```python
from build123d import *

# Parameters (mm, degrees)
SKETCH1_W           = 27.5
SKETCH1_H           = 32.4
BOSS_EXTRUDE1_DEPTH = 1.6
SKETCH2_W           = 18.4
SKETCH2_H           = 13.4
BOSS_EXTRUDE2_DEPTH = 9.5
SKETCH3_W           = 31.3
SKETCH3_H           = 19.46
BOSS_EXTRUDE3_DEPTH = 2.55
SKETCH6_W           = 3
SKETCH6_H           = 13.4
CUT_EXTRUDE1_DEPTH  = 2.54
CUT_EXTRUDE2_DEPTH  = 2.54
SKETCH9_W           = 31.3
SKETCH9_H           = 2.55
BOSS_EXTRUDE4_DEPTH = 2.132
SKETCH11_W          = 31.3
SKETCH11_H          = 26.3172
BOSS_EXTRUDE5_DEPTH = 8
SKETCH12_W          = 20.25
SKETCH12_H          = 1.678
CUT_EXTRUDE3_DEPTH  = 8
FILLET1_R           = 0.5
SKETCH13_R          = 1.45
CUT_EXTRUDE4_DEPTH  = 6
FILLET2_R           = 3.75
FILLET3_R           = 3.75
FILLET4_R           = 3.75
FILLET5_R           = 3.75
FILLET6_R           = 3.75
FILLET7_R           = 3.75
FILLET8_R           = 3.75
FILLET9_R           = 3.75


# Some blends are built 0.0001 mm under size
with BuildPart() as part:
    # Sketch1 → Boss-Extrude1 (new body)
    with BuildSketch(Plane.XY):
        with Locations((-13.75, 16.2)):
            Rectangle(SKETCH1_W, SKETCH1_H)
    extrude(amount=BOSS_EXTRUDE1_DEPTH)

    # Sketch2 → Boss-Extrude2 (add)
    with BuildSketch(Plane.XY.offset(1.6)):
        with Locations((-13.75, 37.1)):
            Rectangle(SKETCH2_W, SKETCH2_H)
    extrude(amount=BOSS_EXTRUDE2_DEPTH)

    # Sketch3 → Boss-Extrude3 (add)
    with BuildSketch(Plane(origin=(0, 0, 0), x_dir=(-1, 0, 0), z_dir=(0, 0, -1))):
        with Locations((13.75, -7.73)):
            Rectangle(SKETCH3_W, SKETCH3_H)
    extrude(amount=BOSS_EXTRUDE3_DEPTH)

    # Sketch6 → Cut-Extrude1 (cut)
    with BuildSketch(Plane.XY.offset(11.1)):
        with Locations((-17.56, 37.1)):
            Rectangle(SKETCH6_W, SKETCH6_H)
        with Locations((-9.94, 37.1)):
            Rectangle(SKETCH6_W, SKETCH6_H)
    extrude(amount=-CUT_EXTRUDE1_DEPTH, mode=Mode.SUBTRACT)

    # Sketch7 → Cut-Extrude2 (cut)
    with BuildSketch(Plane.XY.offset(11.1)):
        with BuildLine():
            Line((-8.44, 40.9552), (-8.44, 42.830691669))
            ThreePointArc((-8.44, 42.830691669), (-9.566358689, 42.178465098), (-10.011, 40.9552))
            Line((-10.011, 40.9552), (-8.44, 40.9552))
        make_face()
        with BuildLine():
            Line((-8.44, 39.079708331), (-8.44, 40.9552))
            Line((-8.44, 40.9552), (-10.011, 40.9552))
            ThreePointArc((-10.011, 40.9552), (-9.566358689, 39.731934902), (-8.44, 39.079708331))
        make_face()
        with BuildLine():
            ThreePointArc((-6.201, 40.9552), (-6.758961582, 42.302238418), (-8.106, 42.8602))
            Line((-8.106, 42.8602), (-8.106, 40.9552))
            Line((-8.106, 40.9552), (-6.201, 40.9552))
        make_face()
        with BuildLine():
            Line((-6.201, 40.9552), (-8.106, 40.9552))
            Line((-8.106, 40.9552), (-8.106, 39.0502))
            ThreePointArc((-8.106, 39.0502), (-6.758961582, 39.608161582), (-6.201, 40.9552))
        make_face()
        with BuildLine():
            Line((-8.106, 40.9552), (-8.106, 42.8602))
            ThreePointArc((-8.106, 42.8602), (-8.273650486, 42.852808578), (-8.44, 42.830691669))
            Line((-8.44, 42.830691669), (-8.44, 40.9552))
            Line((-8.44, 40.9552), (-8.106, 40.9552))
        make_face()
        with BuildLine():
            Line((-8.106, 39.0502), (-8.106, 40.9552))
            Line((-8.106, 40.9552), (-8.44, 40.9552))
            Line((-8.44, 40.9552), (-8.44, 39.079708331))
            ThreePointArc((-8.44, 39.079708331), (-8.273650486, 39.057591422), (-8.106, 39.0502))
        make_face()
    extrude(amount=-CUT_EXTRUDE2_DEPTH, mode=Mode.SUBTRACT)

    # Sketch9 → Boss-Extrude4 (add)
    with BuildSketch(Plane.XZ.offset(17.46)):
        with Locations((-13.75, -1.275)):
            Rectangle(SKETCH9_W, SKETCH9_H)
    extrude(amount=BOSS_EXTRUDE4_DEPTH)

    # Sketch11 → Boss-Extrude5 (add)
    with BuildSketch(Plane.XZ.offset(19.592)):
        with Locations((-13.75, 10.6086)):
            Rectangle(SKETCH11_W, SKETCH11_H)
    extrude(amount=BOSS_EXTRUDE5_DEPTH)

    # Sketch12 → Cut-Extrude3 (cut)
    with BuildSketch(Plane.XZ.offset(27.592)):
        with Locations((-13.75, 21.609)):
            Rectangle(SKETCH12_W, SKETCH12_H)
    extrude(amount=-CUT_EXTRUDE3_DEPTH, mode=Mode.SUBTRACT)

    # Fillet1
    fillet1_edges = [part.edges().sort_by_distance(p)[0] for p in [
        (-23.875, -27.592, 21.609),
        (-13.75, -27.592, 20.77),
        (-3.625, -27.592, 21.609),
        (-13.75, -27.592, 22.448),
    ]]
    fillet(fillet1_edges, radius=FILLET1_R)

    # Sketch13 → Cut-Extrude4 (cut)
    with BuildSketch(Plane.XY.offset(23.7672)):
        with Locations((-19.7549, -23.592)):
            Circle(SKETCH13_R)
        with Locations((-7.7451, -23.592)):
            Circle(SKETCH13_R)
    extrude(amount=-CUT_EXTRUDE4_DEPTH, mode=Mode.SUBTRACT)

    # Fillet2
    fillet2_edges = [part.edges().sort_by_distance(p)[0] for p in [
        (-13.75, -19.592, 0),
    ]]
    fillet(fillet2_edges, radius=FILLET2_R)

    # Fillet3
    # the kernel refuses this fillet: 3.75 mm, written as the material it adds along each edge
    with BuildSketch(Plane(origin=(0, 2, 0), x_dir=(0, 0, -1), z_dir=(-1, 0, 0))) as fillet3_piece_1:
        with BuildLine():
            CenterArc((3.75, -3.552815785), FILLET3_R, 108.662924885, 71.337075115)
            Line((0, -3.552815785), (0, 0))
            Line((0, 0), (2.55, 0))
        make_face()
    extrude(amount=27.5)

    # Fillet4
    fillet4_edges = [part.edges().sort_by_distance(p)[0] for p in [
        (-13.75, 30.4, 1.6),
    ]]
    fillet(fillet4_edges, radius=FILLET4_R)

    # Fillet5
    fillet5_edges = [part.edges().sort_by_distance(p)[0] for p in [
        (-22.95, 29.525, 1.6),
    ]]
    fillet(fillet5_edges, radius=FILLET5_R)

    # Fillet6
    fillet6_edges = [part.edges().sort_by_distance(p)[0] for p in [
        (-4.55, 29.525, 1.6),
    ]]
    fillet(fillet6_edges, radius=FILLET6_R)

    # Fillet7
    fillet7_edges = [part.edges().sort_by_distance(p)[0] for p in [
        (-22.95, 32.4, 3.475),
    ]]
    fillet(fillet7_edges, radius=FILLET7_R - 0.0001)  # a hair under: the kernel refuses the full size

    # Fillet8
    fillet8_edges = [part.edges().sort_by_distance(p)[0] for p in [
        (-4.55, 32.4, 3.475),
    ]]
    fillet(fillet8_edges, radius=FILLET8_R - 0.0001)  # a hair under: the kernel refuses the full size

    # Fillet9
    # the kernel refuses this fillet: 3.75 mm, written as the material it adds along each edge
    with BuildSketch(Plane(origin=(0, 2, 0), x_dir=(1, 0, 0), z_dir=(0, 0, -1))) as fillet9_piece_1_section:
        with BuildLine():
            CenterArc((3.75, -3.261901286), FILLET9_R, 119.559908379, 60.440091621)
            Line((0, -3.261901286), (0, 0))
            Line((0, 0), (1.9, 0))
        make_face()
    fillet9_piece_1 = extrude(amount=2.55, mode=Mode.PRIVATE)
    fillet9_piece_1 = fillet9_piece_1 - Plane(origin=(1.353199259, 5.552815785, -3.75), x_dir=(0, 0, -1), z_dir=(1, 0, 0)) * Cylinder(3.75, 19, mode=Mode.PRIVATE)
    add(fillet9_piece_1)
    with BuildSketch(Plane(origin=(-27.5, 2, 0), x_dir=(0, 1, 0), z_dir=(0, 0, -1))) as fillet9_piece_2_section:
        with BuildLine():
            CenterArc((3.261901286, -3.75), FILLET9_R, 90, 60.440091621)
            Line((0, -1.9), (0, 0))
            Line((0, 0), (3.261901286, 0))
        make_face()
    fillet9_piece_2 = extrude(amount=2.55, mode=Mode.PRIVATE)
    fillet9_piece_2 = fillet9_piece_2 - Plane(origin=(-28.00314891, 5.552815785, -3.75), x_dir=(0, 0, -1), z_dir=(1, 0, 0)) * Cylinder(3.75, 19, mode=Mode.PRIVATE)
    add(fillet9_piece_2)


solid = part.part
```
Could you check a few things on this model? Use its own coordinates, in mm. A direction names the side the tool comes from. Round coordinates to 2 decimals unless told otherwise and drop trailing zeros. Loops run counter-clockwise (first coordinate to the right, second up) from the corner with the lowest first, then second, coordinate; pieces in that order, holes last. Notation, with made-up numbers: M -5,65 L 21,65 A26 ccw 21,91 Z; hole C 59,81.25 d7. An arc over 180 degrees is marked long. Put each result on its own line as item: value.
Q1. Imagine slicing it at D-D (y = -2.5). Write out the boundary of the cut face in (x, z), then the cut area to 3 significant figures.
Check result:
outline: M -29.4,-2.55 L 1.9,-2.55 L 1.9,0 L -29.4,0 Z
area: 79.8 mm2
Q2. For pin 1 (12 mm diameter, centred on y = 28.5, z = 21, fed in from -X); pin 2 (1.9 mm diameter, centred on x = -6, y = 39.5, fed in from +Z); pin 3 (1 mm diameter, centred on y = 15.5, z = 1.5, fed in from +X); pin 4 (5 mm diameter, centred on x = -18.5, z = 18.5, fed in from +Y), each with a flat end and sliding along its axis, tell me the tip position at first contact or that it passes through.
Check result:
pin 1: through
pin 2: z = 11.1
pin 3: x = 0
pin 4: y = -19.59
Q3. Imagine slicing it at C-C (z = 4.5). Write out the boundary of the cut face in (x, y), then the cut area to 3 significant figures.
Check result:
outline: M -29.4,-27.59 L 1.9,-27.59 L 1.9,-19.59 L -29.4,-19.59 Z; M -23.05,30.3 L -4.45,30.3 L -4.45,35.3 A3.75 cw -4.55,36.15 L -4.55,43.8 L -22.95,43.8 L -22.95,36.15 A3.75 cw -23.05,35.3 Z
area: 500 mm2
Q4. Imagine slicing it at B-B (x = -10). Write out the boundary of the cut face in (y, z), then the cut area to 3 significant figures.
Check result:
outline: M -27.59,-2.55 L 2,-2.55 A3.75 cw 5.55,0 L 32.4,0 L 32.4,1.6 L 43.8,1.6 L 43.8,8.56 L 30.4,8.56 L 30.4,5.35 A3.75 cw 26.65,1.6 L 0,1.6 L 0,0 L -15.84,0 A3.75 cw -19.59,3.75 L -19.59,20.77 L -27.09,20.77 A0.5 ccw -27.59,20.27 Z; M -27.59,22.95 A0.5 ccw -27.09,22.45 L -19.59,22.45 L -19.59,23.77 L -27.59,23.77 Z
area: 406 mm2
Q5. On a 3-axis mill with a long thin cutter (end or side, diameter ignored), from which of +Z, -Z, +X, -X, +Y, -Y can I reach the whole of each face in a straight line? I mean faces 1 (the face through (-14, -19.592, 14)), 2 (the face through (-18, 37, 8.56)), 3 (the face through (-23.875, -23, 22)), 4 (the face through (-8, -24, 17.767)), 5 (the face through (-14, 19, 0)). Say none if no direction works.
Check result:
face 1: +Z, +X, -X
face 2: +Z, +Y
face 3: +Y, -Y
face 4: +Z
face 5: -Z, +X, -X, +Y
Q6. Thinking about a two-plate mould opening in Y: for faces 6 (the face through (-4.216, 34.603, 2.668)), 7 (the face through (-20.1, -25, 19.3)), 8 (the face through (-14, -23, 20.77)), which applies, released by +Y, released by -Y, zero draft, split by the parting line, or undercut?
Check result:
face 6: released by +Y
face 7: undercut
face 8: zero draft
Q7. Imagine slicing it at A-A (z = 10). Write out the boundary of the cut face in (x, y) (3 decimals), then the cut area to 3 significant figures.
Check result:
outline: M -29.4,-27.592 L 1.9,-27.592 L 1.9,-19.592 L -29.4,-19.592 Z; M -22.95,30.4 L -19.06,30.4 L -19.06,43.8 L -22.95,43.8 Z; M -16.06,30.4 L -11.44,30.4 L -11.44,43.8 L -16.06,43.8 Z; M -8.44,30.4 L -4.55,30.4 L -4.55,43.8 L -8.44,43.8 L -8.44,42.831 A1.905 cw long -8.44,39.08 Z
area: 410 mm2
Q8. I need wall thicknesses on probe 1 along Y at (x, z) = (-5, 8.25); probe 2 along Z at (x, y) = (-15.5, -20); probe 3 along Y at (x, z) = (0, 4.5). Which ranges of each line are inside material? Lowest first, please.
Check result:
probe 1: -27.59 to -19.59, 30.4 to 43.8
probe 2: -2.55 to 20.77, 22.45 to 23.77
probe 3: -27.59 to -19.59
